Source: three-view drawing plus pictorial views. Frame: mm from the lowest corner of the part. A direction names the side the tool comes from. Give positions to 0.01 mm unless a question says otherwise; leave off trailing zeros. Loops run counter-clockwise (first coordinate to the right, second up) from the corner with the lowest first, then second, coordinate; pieces in that order, holes last. Notation, with made-up numbers: (-12, 56) - (20, 56) arc R7 ccw to (20, 63) - close; hole circle Ø11 at (32.25, 34). An arc over 180 degrees is marked (long way). Put each result on its own line as item: value.
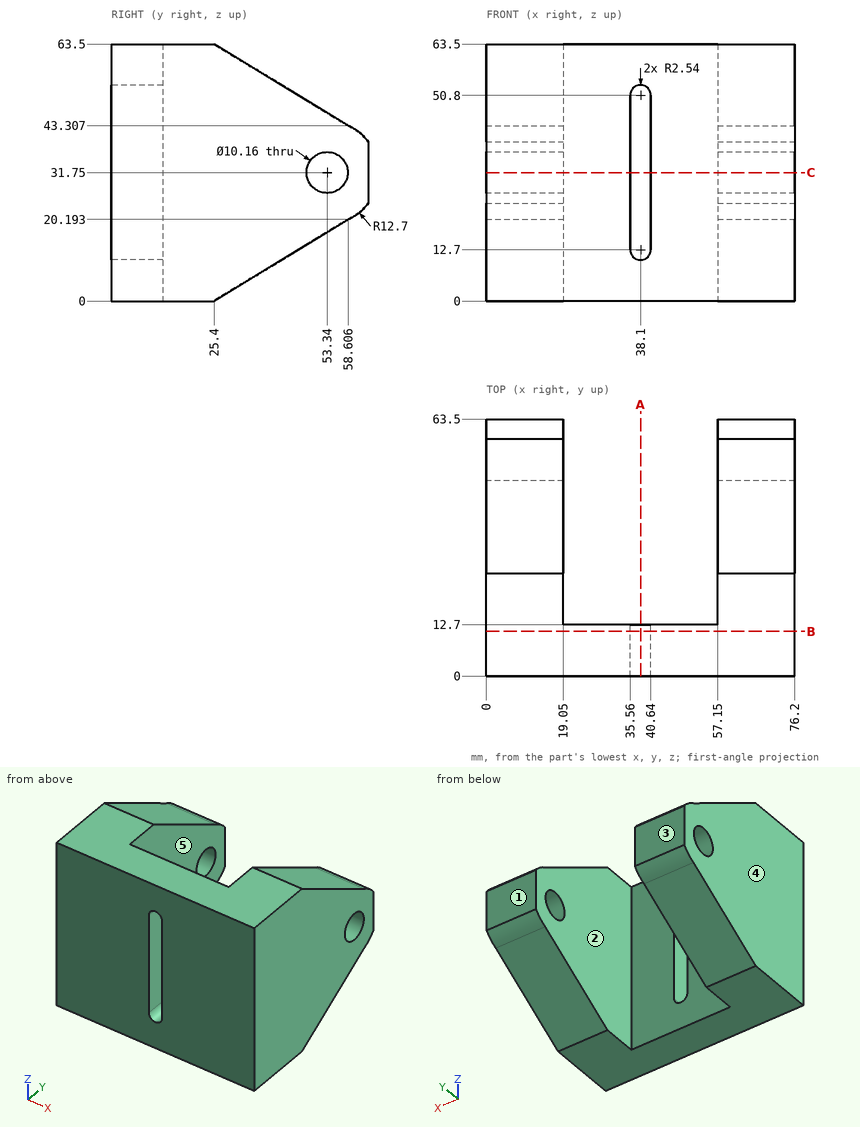
1) Section query B-B, the plane y = 11. Output: boundary loops of the cut face in (x, z), plus the area to 4 significant figures.
Check result:
outline: (0, 0) - (76.2, 0) - (76.2, 63.5) - (0, 63.5) - close; hole (35.56, 12.7) arc R2.54 ccw to (40.64, 12.7) - (40.64, 50.8) arc R2.54 ccw to (35.56, 50.8) - close
area: 4,625 mm²
2) Pin query (flat end, axial travel): P1, Ø2, axis at x = 53, z = 53, coming from the +Y side. Return the tip coordinate at first contact, or that it passes through.
Check result:
P1: y = 12.7
3) Mould query, pull axis X, two halves, no side actions, for the marked faces 3, 4 and 5. Classes: pulls with the +X half, pulls with the -X half, needs draft (parallel to the pull), parting line crosses it, or undercut.
Check result:
face 3: needs draft
face 4: pulls with the -X half
face 5: undercut
4) Section query A-A, the plane x = 38.1. Output: boundary loops of the cut face in (y, z), plus the area to 3 significant figures.
Check result:
outline: (0, 0) - (12.7, 0) - (12.7, 10.16) - (0, 10.16) - close; (0, 53.34) - (12.7, 53.34) - (12.7, 63.5) - (0, 63.5) - close
area: 258 mm²
5) Access query for the marked faces 1 and 2. Directions: +Z, -Z, +X, -X, +Y, -Y. A direction counts if a zero-diameter tool reaches every point of the face in a straight line with its end or side. Return the directions, or none.
Check result:
face 1: +Z, -Z, +X, -X, +Y
face 2: +Z, -Z, +Y
6) Section query C-C, the plane z = 31.75. Output: boundary loops of the cut face in (x, y).
Check result:
outline: (0, 0) - (35.56, 0) - (35.56, 12.7) - (19.05, 12.7) - (19.05, 48.26) - (0, 48.26) - close; (0, 58.42) - (19.05, 58.42) - (19.05, 63.5) - (0, 63.5) - close; (40.64, 0) - (76.2, 0) - (76.2, 48.26) - (57.15, 48.26) - (57.15, 12.7) - (40.64, 12.7) - close; (57.15, 58.42) - (76.2, 58.42) - (76.2, 63.5) - (57.15, 63.5) - close
7) Material intervals for line 1 along Y through (x, z) = (10.5, 31.75); line 2 along X through (y, z) = (4, 21); line 3 along X through (y, z) = (18, 7), sorted ascending. Write a range as [from, to].
Check result:
line 1: [0, 48.26], [58.42, 63.5]
line 2: [0, 35.56], [40.64, 76.2]
line 3: [0, 19.05], [57.15, 76.2]
